Source: CAD feature listing. Evaluate the final solid. Frame: model axes, mm. A direction names the side the tool comes from. Give positions to 0.01 mm unless a question says otherwise; leave off trailing zeros. Order: outer loops, then holes, each group sorted by start corner. A loop starts at its lowest first (then second) coordinate and runs counter-clockwise, first axis right, second up. Notation, with made-up numbers: M 47,-34.75 L 66,-34.75 A8 cw 66,-21.75 Z; hole C 32,-11 d9. An arc over 180 degrees is marked long. Answer as a JSON object with one key per item and string values. Group by question number.
1. Material intervals for L1, parallel to X at y = 0.65, z = 6; L2, parallel to Z at x = 0, y = 4; L3, parallel to Y at x = 1.6, z = -9.5, sorted ascending. Write a range as [from, to].
2. Section query B-B (y = 7.25). Output: boundary loops of the cut face in (x, z), plus the area to 3 significant figures.
3. Pull-direction query (X, two-part tool) for faces 3 (the flat face through (0, 5, -12)), 4 (the cylindrical face through (0, 6, 11)), 5 (the cylindrical face through (-2.14, 9.1, 10.99)); classes: +X half, -X half, draft (parallel to the pull), parting line (faces both ways), or undercut.
4. Pin query (flat end, axial travel): P1, Ø2.5, axis at x = 0, y = 7.5, coming from the -Z side; P2, Ø3, axis at x = 0.5, z = 1, coming from the +Y side. Return the tip coordinate at first contact, or that it passes through.
5. Section query C-C (x = -1.25). Output: boundary loops of the cut face in (y, z), plus the area to 3 significant figures.
6. Section query A-A (z = 6). Output: boundary loops of the cut face in (x, y).
7. Section query D-D (x = 2.2). Output: boundary loops of the cut face in (y, z), plus the area to 4 significant figures.
8. Set-up query: faces 1 (the flat face through (0, 5, -10)), 2 (the cylindrical face through (0.04, 0.6, 11.43)). Return all of +Z, -Z, +X, -X, +Y, -Y with unobstructed straight access to the full face (end or side cutting, diameter ignored); none if empty.
Autodesk Inventor part; units mm, degrees
ref_plane "YZ Plane" through (0, 0, 0) normal (1, 0, 0) x (0, 1, 0)
ref_plane "XZ Plane" through (0, 0, 0) normal (0, 1, 0) x (-1, 0, 0)
ref_plane "XY Plane" through (0, 0, 0) normal (0, 0, 1) x (1, 0, 0)
sketch "スケッチ2" plane through (0, 0, 0) normal (0, 1, 0) x (-1, 0, 0)
  line L0 (3, 12) -> (-3, 12)
  line L1 (-3, 12) -> (-3, -12)
  line L2 (-3, -12) -> (3, -12)
  line L3 (3, -12) -> (3, 12)
  line L4 (3, 12) -> (-3, -12) construction
  line L5 (-3, 12) -> (3, -12) construction
  point P0 (0, 0)
  dimension "d0" = 6
  dimension "d1" = 24
extrude "押し出し1" add sketch "スケッチ2" along normal blind 2
sketch "スケッチ3" plane through (0, 2, 0) normal (0, 1, 0) x (1, 0, 0)
  line L0 (0, 0) -> (17.0927, 0) construction
  circle A0 centre (0, -6) radius 1.5
  circle A1 centre (0, 6) radius 1.5
  dimension "d25" = 3
extrude "押し出し2" cut sketch "スケッチ3" against normal through all
sketch "スケッチ4" plane through (0, 2, 0) normal (0, 1, 0) x (1, 0, 0)
  line L0 (-3, -12) -> (3, -12)
  line L1 (3, -12) -> (-3, -12)
  line L2 (-3, -12) -> (-3, -10)
  line L3 (-3, -10) -> (3, -10)
  line L4 (3, -10) -> (3, -12)
  line L5 (0, 0) -> (11.7228, 0) construction
  line L6 (-3, 12) -> (3, 12)
  line L7 (-3, 12) -> (-3, 10)
  line L8 (-3, 10) -> (3, 10)
  line L9 (3, 10) -> (3, 12)
  dimension "d8" = 6
  dimension "d9" = 2
extrude "押し出し3" add sketch "スケッチ4" along normal blind 8
sketch "スケッチ6" plane through (-3, 0, 12) normal (0, 0, 1) x (1, 0, 0)
  circle A0 centre (3, 7.5) radius 1.5
  point P0 (3, 0)
  dimension "d36" = 3
extrude "押し出し4" cut sketch "スケッチ6" against normal through all
fillet "フィレット1" radius 2 1 edges at (0, 0, 12)
fillet "フィレット2" radius 0.5 1 edges at (0, 2, 10)
fillet "フィレット3" radius 0.5 1 edges at (0, 2, -10)
fillet "フィレット4" radius 2 1 edges at (0, 0, -12)
fillet "フィレット5" radius 3 4 edges at (3, 10, 11) (-3, 10, 11) (3, 10, -11) (-3, 10, -11)
properties part number "Plasma Box Hinge"
Answer sheet:
{
 "1": {"L1": "[-3, -1.5], [1.5, 3]", "L2": "[-12, -10], [10, 12]", "L3": "[0, 2]"},
 "2": {"outline": "M -2.99,-12 L -1.48,-12 L -1.48,-10 L -2.99,-10 Z; M -2.99,10 L -1.48,10 L -1.48,12 L -2.99,12 Z; M 1.48,-12 L 2.99,-12 L 2.99,-10 L 1.48,-10 Z; M 1.48,10 L 2.99,10 L 2.99,12 L 1.48,12 Z", "area": "12.1 mm^2"},
 "3": {"face 3": "draft", "face 4": "undercut", "face 5": "-X half"},
 "4": {"P1": "through", "P2": "y = 2"},
 "5": {"outline": "M 0,-10 A2 ccw 2,-12 L 6.67,-12 L 6.67,-10 L 2.5,-10 A0.5 cw 2,-9.5 L 2,-6.83 L 0,-6.83 Z; M 0,-5.17 L 2,-5.17 L 2,5.17 L 0,5.17 Z; M 0,6.83 L 2,6.83 L 2,9.5 A0.5 cw 2.5,10 L 6.67,10 L 6.67,12 L 2,12 A2 ccw 0,10 Z; M 8.33,-12 L 9.73,-12 L 9.73,-10 L 8.33,-10 Z; M 8.33,10 L 9.73,10 L 9.73,12 L 8.33,12 Z", "area": "64.0 mm^2"},
 "6": {"outline": "M -3,0 L -1.5,0 L -1.5,2 L -3,2 Z; M 1.5,0 L 3,0 L 3,2 L 1.5,2 Z"},
 "7": {"outline": "M 0,-10 A2 ccw 2,-12 L 9.04,-12 L 9.04,-10 L 2.5,-10 A0.5 cw 2,-9.5 L 2,9.5 A0.5 cw 2.5,10 L 9.04,10 L 9.04,12 L 2,12 A2 ccw 0,10 Z", "area": "74.55 mm^2"},
 "8": {"face 1": "+X, -X, +Y", "face 2": "+Z, +X, -X, -Y"}
}
